Verification items for the finished model (mm, model axes). A direction names the side the tool comes from. Round coordinates to 2 decimals unless told otherwise and drop trailing zeros. Order: outer loops, then holes, each group sorted by start corner. A loop starts at its lowest first (then second) coordinate and runs counter-clockwise, first axis right, second up. Notation, with made-up numbers: M 83.25,60.25 L 134.25,60.25 A20 cw 134.25,95.25 Z; hole C 27,-3.75 d11. An arc over 180 degrees is marked long. Use one line per item in the form item = value. Start each with the question number.
Item 1: Tool access check on faces 4 (the flat face through (-28, 45, 39)), 5 (the flat face through (-15.9, 45.5, 0)). Record the directions out of +Z, -Z, +X, -X, +Y, -Y that give a thin tool (end or side, any length) a straight path to the whole face; none if there is none.
Item 2: Cross-section at C-C on x = -14. Enter the section's corners in (y, z).
Item 3: Release check for a two-part mould opening along Y. For faces 1 (the flat face through (-25, 50, 39)), 2 (the flat face through (0, 30, 39)), 3 (the cylindrical face through (-2.54, 27.54, 36.14)) record: +Y half, -Y half, draft (parallel to the pull), parting line (faces both ways), or undercut.
Item 4: Cross-section at D-D on z = 55.5. Enter the section's corners in (x, y), then the cut area to 3 significant figures.
Item 5: Cross-section at A-A on z = 40. Enter the section's corners in (x, y).
Item 6: Cross-section at B-B on y = 22.5. Enter the section's corners in (x, z), then the cut area to 4 significant figures.
Item 7: Thickness scan on probe 1 along Z at (x, y) = (-3, 22); probe 2 along Y at (x, z) = (-29.5, 65.5); probe 3 along X at (y, z) = (34, 27). Record the ranges inside material, lowest first. Write a range as [from, to].
Item 8: Go/stop test with flat-tipped pins: pin 1 Ø13.5 at (x, z) = (-20, 30) entering from -Y; pin 2 Ø10 at (y, z) = (22.5, 40) entering from +X; pin 3 Ø5 at (y, z) = (8.5, 61) entering from -X. Record where each tip stops, or that it passes through.
from build123d import *

# Parameters (mm, degrees)
SALIENTE_EXTRUIR1_DEPTH = 80
CORTAR_EXTRUIR1_REACH   = 106.523
CROQUIS2_R              = 6.35


with BuildPart() as part:
    # Croquis1 → Saliente-Extruir1 (new body)
    with BuildSketch(Plane.XY):
        Polygon((0, 0), (0, 50), (-50, 50), (-50, 45), (-5, 45), (-5, 0), align=None)
    extrude(amount=SALIENTE_EXTRUIR1_DEPTH)

    # Croquis2 → Cortar-Extruir1 (cut, up to next)
    with BuildSketch(Plane.ZY.offset(5), mode=Mode.PRIVATE) as cortar_extruir1_sk1:
        with Locations(Location((40, 22.5, 0), (0, 0, 270))):
            Circle(CROQUIS2_R)
    cortar_extruir1_tool1 = extrude(cortar_extruir1_sk1.sketch, amount=-CORTAR_EXTRUIR1_REACH, mode=Mode.PRIVATE) & part.part
    add(cortar_extruir1_tool1.solids().sort_by_distance((-5, 22.5, 40))[0], mode=Mode.SUBTRACT)


solid = part.part
Output values:
q1.face_4 = +Z, -Z, -X, -Y
q1.face_5 = -Z, +X, -X, +Y, -Y
q2.outline = M 45,0 L 50,0 L 50,80 L 45,80 Z
q3.face_1 = +Y half
q3.face_2 = draft
q3.face_3 = undercut
q4.outline = M -50,45 L -5,45 L -5,0 L 0,0 L 0,50 L -50,50 Z
q4.area = 475 mm2
q5.outline = M -50,45 L -5,45 L -5,28.85 L 0,28.85 L 0,50 L -50,50 Z; M -5,0 L 0,0 L 0,16.15 L -5,16.15 Z
q6.outline = M -5,0 L 0,0 L 0,33.65 L -5,33.65 Z; M -5,46.35 L 0,46.35 L 0,80 L -5,80 Z
q6.area = 336.5 mm2
q7.probe_1 = [0, 33.67], [46.33, 80]
q7.probe_2 = [45, 50]
q7.probe_3 = [-5, 0]
q8.pin_1 = 45
q8.pin_2 = through
q8.pin_3 = -5
